Could you check a few things on this drawing? It's one solid part, dimensions in mm from its lowest x, y, z. Give positions to 0.01 mm unless a question says otherwise; leave off trailing zeros. Loops run counter-clockwise (first coordinate to the right, second up) from the corner with the lowest first, then second, coordinate; pieces in that order, holes last. Notation, with made-up numbers: M 21.25,18.5 L 76.25,18.5 A20 ccw 76.25,22.5 Z; hole C -11.75,59 d9. An arc over 180 degrees is marked long. Answer in a Markdown table with one row per item. Add a question column.
1. I'm going to push flat-ended pins straight in: pin 1 Ø5 at (x, y) = (12.5, 4.5) entering from -Z; pin 2 Ø0.5 at (x, z) = (11, 2) entering from -Y; pin 3 Ø1 at (x, z) = (11, 1) entering from +Y. Where does each tip first touch, or does it pass through?
2. If we section it at A-A on y = 8: List the corners of the cut face in (x, z) for me, then the cut area to 3 significant figures.
3. I need wall thicknesses on line 1 along Y through (x, z) = (1.11, 14.35); line 2 along Z through (x, y) = (17.5, 3.75). Which ranges of each line are inside material? Lowest first, please. Write a range as from..to.
4. If we section it at B-B on x = 2.5: List the corners of the cut face in (y, z) for me, then the cut area to 3 significant figures.
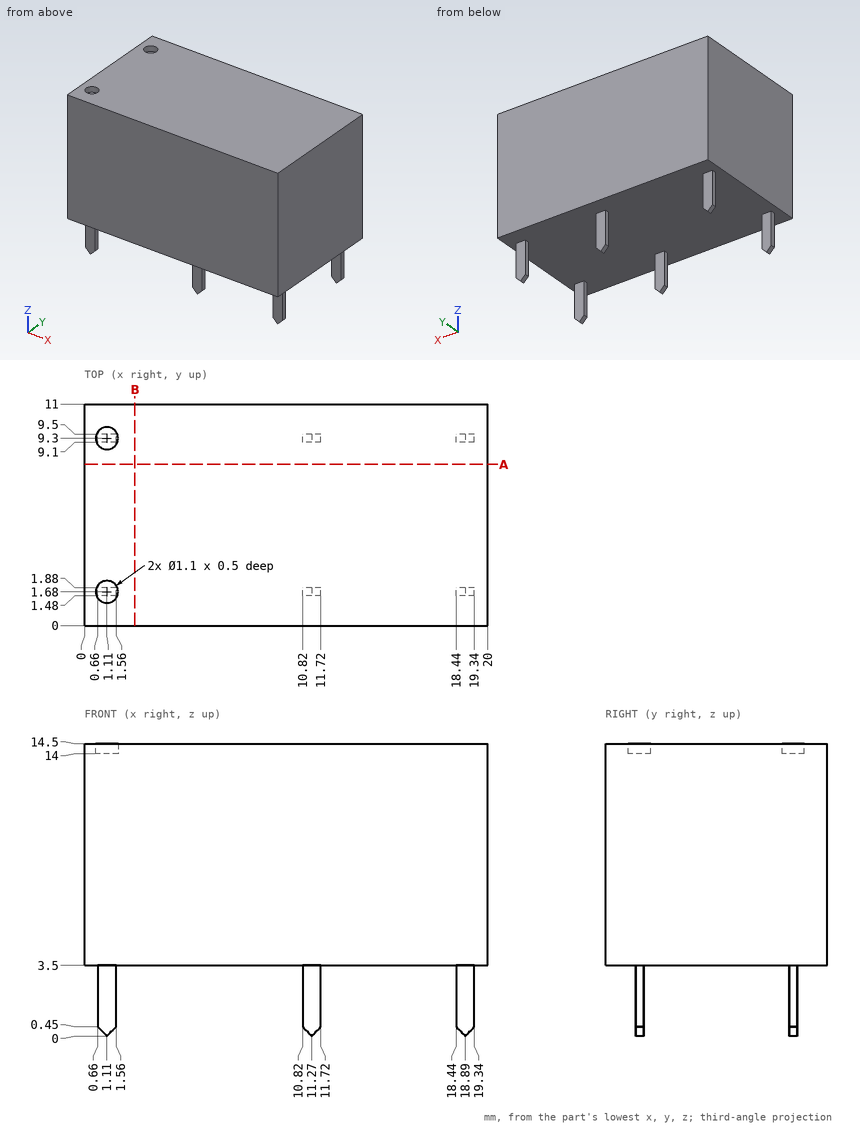
Results:
| question | item | result |
|---|---|---|
| 1 | pin 1 | z = 3.5 |
| 1 | pin 2 | y = 1.48 |
| 1 | pin 3 | y = 9.5 |
| 2 | outline | M 0,3.5 L 20,3.5 L 20,14.5 L 0,14.5 Z |
| 2 | area | 220 mm2 |
| 3 | line 1 | 0..1.13, 2.23..8.75, 9.85..11 |
| 3 | line 2 | 3.5..14.5 |
| 4 | outline | M 0,3.5 L 11,3.5 L 11,14.5 L 0,14.5 Z |
| 4 | area | 121 mm2 |
